Design review of the part built by this model. Coordinates are the model's own, in mm. Round coordinates to 2 decimals unless told otherwise and drop trailing zeros. Order: outer loops, then holes, each group sorted by start corner. A loop starts at its lowest first (then second) coordinate and runs counter-clockwise, first axis right, second up. Notation, with made-up numbers: (75, 4) - (131, 4) arc R15 cw to (131, 14) - close; hole circle Ø3 at (-13.5, 43.25). An arc over 180 degrees is marked (long way). Write item = value, one per line.
from build123d import *

# Parameters (mm, degrees)
SKETCH_1_W      = 20
SKETCH_1_H      = 91
SKETCH_1_R      = 1.6
EXTRUDE_1_DEPTH = 1
CHAMFER_1_SIZE  = 2


with BuildPart() as part:
    # 草图1 → 凸台-拉伸1 (new body)
    with BuildSketch(Plane.XY):
        Rectangle(SKETCH_1_W, SKETCH_1_H)
        with Locations((7, 25.5)):
            Circle(SKETCH_1_R, mode=Mode.SUBTRACT)
        with Locations((7, 17.5)):
            Circle(SKETCH_1_R, mode=Mode.SUBTRACT)
        with Locations((7, -14.5)):
            Circle(SKETCH_1_R, mode=Mode.SUBTRACT)
        with Locations((7, -22.5)):
            Circle(SKETCH_1_R, mode=Mode.SUBTRACT)
    extrude(amount=EXTRUDE_1_DEPTH)

    # 倒角1
    chamfer_1_edges = [part.edges().sort_by_distance(p)[0] for p in [
        (10, -45.5, 0.5),
        (-10, -45.5, 0.5),
        (-10, 45.5, 0.5),
        (10, 45.5, 0.5),
    ]]
    chamfer(chamfer_1_edges, length=CHAMFER_1_SIZE)


solid = part.part
Item 1: Take a section at C-C, the plane z = 0.2. State the section outline as (x, y) points, and give its area (3 significant figures).
Data:
outline = (-10, -43.5) - (-8, -45.5) - (8, -45.5) - (10, -43.5) - (10, 43.5) - (8, 45.5) - (-8, 45.5) - (-10, 43.5) - close; hole circle Ø3.2 at (7, -22.5); hole circle Ø3.2 at (7, -14.5); hole circle Ø3.2 at (7, 17.5); hole circle Ø3.2 at (7, 25.5)
area = 1,780 mm2
Item 2: The part is to be moulded in two halves that separate along X. For faces 1 (the face through (0, 1, 0)), 2 (the face through (5.73, 24.53, 0.49)), 3 (the face through (5.82, -13.42, 0.49)), 4 (the face through (-9, 44.5, 0.5)), say which applies: +X half, -X half, draft (parallel to the pull), parting line (faces both ways), or undercut.
Data:
face_1 = draft
face_2 = undercut
face_3 = undercut
face_4 = -X half
Item 3: Take a section at A-A, the plane y = 17.5. State the section outline as (x, z) points, and give its area (3 significant figures).
Data:
outline = (-10, 0) - (5.4, 0) - (5.4, 1) - (-10, 1) - close; (8.6, 0) - (10, 0) - (10, 1) - (8.6, 1) - close
area = 16.8 mm2
Item 4: Take a section at B-B, the plane x = 7. State the section outline as (y, z) points, and give its area (3 significant figures).
Data:
outline = (-45.5, 0) - (-24.1, 0) - (-24.1, 1) - (-45.5, 1) - close; (-20.9, 0) - (-16.1, 0) - (-16.1, 1) - (-20.9, 1) - close; (-12.9, 0) - (15.9, 0) - (15.9, 1) - (-12.9, 1) - close; (19.1, 0) - (23.9, 0) - (23.9, 1) - (19.1, 1) - close; (27.1, 0) - (45.5, 0) - (45.5, 1) - (27.1, 1) - close
area = 78.2 mm2
Item 5: For line 1 along Y through (x, z) = (7, 0.7); line 2 along Y through (x, z) = (5.75, 0.25); line 3 along Y through (x, z) = (-8.5, 0.8), list the stretches that pass through material, from the lowest coordinate up. Write a range as [from, to].
Data:
line_1 = [-45.5, -24.1], [-20.9, -16.1], [-12.9, 15.9], [19.1, 23.9], [27.1, 45.5]
line_2 = [-45.5, -23.5], [-21.5, -15.5], [-13.5, 16.5], [18.5, 24.5], [26.5, 45.5]
line_3 = [-45, 45]
